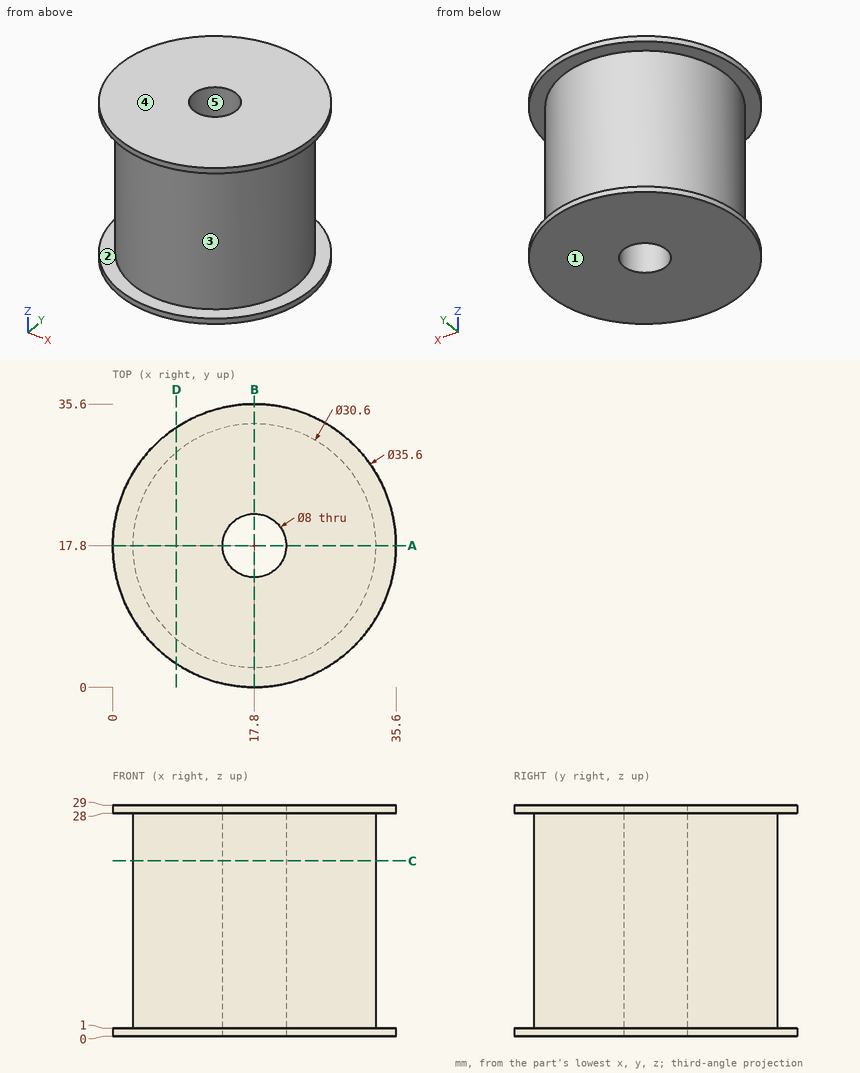
The drawing under review shows one solid part. Ordinate dimensions are in mm from its lowest x, y, z. A direction names the side the tool comes from. Coordinates: 2 decimals unless noted, no trailing zeros. Order: outer loops, then holes, each group sorted by start corner. A loop starts at its lowest first (then second) coordinate and runs counter-clockwise, first axis right, second up. Notation, with made-up numbers: (-36.5, -3) -> (-32.5, -3) arc R11 cw to (-32.5, 13) -> close; hole circle Ø6 at (-25, 40.25). An arc over 180 degrees is marked (long way). One line per item, written item: value.
1) Draft analysis for pull direction Y (two halves, no side actions). For the marked faces 3, 4 and 5, state which applies: +Y half, -Y half, draft (parallel to the pull), parting line (faces both ways), or undercut.
Output values:
face 3: parting line
face 4: draft
face 5: undercut
2) We need section C-C, the plane z = 22. Give the boundary of the cut face in (x, y).
Output values:
outline: circle Ø30.6 at (17.8, 17.8); hole circle Ø8 at (17.8, 17.8)
3) Clearance check with flat-ended pins moving along their axes: P1, Ø6, axis at y = 30.5, z = 23.5, coming from the +X side; P2, Ø6, axis at x = 11, z = 16.5, coming from the +Y side; P3, Ø8, axis at x = 19, z = 6, coming from the -Y side; P4, Ø5, axis at x = 17.8, y = 17.8, coming from the -Z side. State where each tip first meets the part, or that it passes through.
Output values:
P1: stops at x = 29.63
P2: stops at y = 32.62
P3: stops at y = 2.5
P4: passes through
4) We need section D-D, the plane x = 8. Give the boundary of the cut face in (y, z), then the cut area to 3 significant figures.
Output values:
outline: (2.94, 0) -> (32.66, 0) -> (32.66, 1) -> (29.55, 1) -> (29.55, 28) -> (32.66, 28) -> (32.66, 29) -> (2.94, 29) -> (2.94, 28) -> (6.05, 28) -> (6.05, 1) -> (2.94, 1) -> close
area: 694 mm2
5) To check wall thickness, follow probe 1 along Y at (x, z) = (17.8, 7.25); probe 2 along Z at (x, y) = (32, 10.5); probe 3 along X at (y, z) = (14.5, 10.25). State the ranges of each line that lie inside material, in increasing order. Write a range as [from, to].
Output values:
probe 1: y = [2.5, 13.8], [21.8, 33.1]
probe 2: z = [0, 1], [28, 29]
probe 3: x = [2.86, 15.54], [20.06, 32.74]
6) We need section A-A, the plane y = 17.8. Give the boundary of the cut face in (x, z), then the cut area to 3 significant figures.
Output values:
outline: (0, 0) -> (13.8, 0) -> (13.8, 29) -> (0, 29) -> (0, 28) -> (2.5, 28) -> (2.5, 1) -> (0, 1) -> close; (21.8, 0) -> (35.6, 0) -> (35.6, 1) -> (33.1, 1) -> (33.1, 28) -> (35.6, 28) -> (35.6, 29) -> (21.8, 29) -> close
area: 665 mm2
7) Machinability: for the marked faces 1 and 2, which of the approach directions +Z, -Z, +X, -X, +Y, -Y give a long, thin tool a straight path to every point of the face, cutting with its end or side? Answer none if there is none.
Output values:
face 1: -Z, +X, -X, +Y, -Y
face 2: none
